```python
from build123d import *

# Parameters (mm, degrees)
EXTRUSION1_DEPTH           = 2.1
ESQUISSE2_R                = 5.85
EXTRUSION2_DEPTH           = 5.2
ESQUISSE3_R                = 1.75
EXTRUSION3_DEPTH           = 39.762384708
ESQUISSE4_R                = 3.15
EXTRUSION4_DEPTH           = 4
ESQUISSE5_R                = 2.95
EXTRUSION5_DEPTH           = 3.2
CHANFREIN2_SIZE            = 1.2
D_GAGEMENT_M21_D           = 1.8
R_P_TITION_LIN_AIRE1_COUNT = 6
R_P_TITION_LIN_AIRE1_PITCH = 3.2


with BuildPart() as part:
    # Esquisse1 → Extrusion1 (new body)
    with BuildSketch(Plane.XY):
        with BuildLine():
            Line((-0.179008677, 4.246228432), (30.191384159, 5.526556123))
            ThreePointArc((30.191384159, 5.526556123), (37.220312431, -1.486890222), (29.654324486, -7.917293686))
            Line((29.654324486, -7.917293686), (-0.51715736, -4.218417744))
            ThreePointArc((-0.51715736, -4.218417744), (-4.246612828, 0.169645193), (-0.179008677, 4.246228432))
        make_face()
    extrude(amount=EXTRUSION1_DEPTH)

    # Esquisse2 → Extrusion2 (add)
    with BuildSketch(Plane(origin=(0, 0, 0), x_dir=(-1, 0, 0), z_dir=(0, 0, -1))):
        with Locations(Location((-30.475692058, -1.217453739, 0), (0, 0, 180))):
            Circle(ESQUISSE2_R)
    extrude(amount=EXTRUSION2_DEPTH)

    # Esquisse3 → Extrusion3 (cut, through all)
    with BuildSketch(Plane(origin=(0, 0, -5.2), x_dir=(-1, 0, 0), z_dir=(0, 0, -1))):
        with Locations((-30.475692058, -1.217453739)):
            Circle(ESQUISSE3_R)
    extrude(amount=-EXTRUSION3_DEPTH, mode=Mode.SUBTRACT)

    # Esquisse4 → Extrusion4 (cut)
    with BuildSketch(Plane.XY.offset(2.1)):
        with Locations((30.475692058, -1.217453739)):
            Circle(ESQUISSE4_R)
    extrude(amount=-EXTRUSION4_DEPTH, mode=Mode.SUBTRACT)

    # Esquisse5 → Extrusion5 (cut)
    with BuildSketch(Plane(origin=(0, 0, -5.2), x_dir=(-1, 0, 0), z_dir=(0, 0, -1))):
        with Locations((-30.475692058, -1.217453739)):
            Circle(ESQUISSE5_R)
    extrude(amount=-EXTRUSION5_DEPTH, mode=Mode.SUBTRACT)

    # Chanfrein2
    chanfrein2_edges = [part.edges().sort_by_distance(p)[0] for p in [
        (24.625692058, -1.217453739, -5.2),
        (27.325692058, -1.217453739, 2.1),
    ]]
    chamfer(chanfrein2_edges, length=CHANFREIN2_SIZE)

    # D_gagement M21 (through all)
    with Locations(Plane(origin=(-0.55, 0, 2.1), x_dir=(1, 0, 0), z_dir=(0, 0, 1))):
        with Locations((0, 0)):
            d_gagement_m21 = Hole(D_GAGEMENT_M21_D / 2)

    # R_p_tition lin_aire1: D_gagement M21 ×6
    with Locations(*[Vector(0.9992309921094119, -0.0392100039280862, 0) * (i * R_P_TITION_LIN_AIRE1_PITCH) for i in range(1, R_P_TITION_LIN_AIRE1_COUNT)]):
        add(d_gagement_m21, mode=Mode.SUBTRACT)


solid = part.part
```
Input: part model. Units: mm. Frame: model coordinates. A direction names the side the tool comes from. Give positions to 0.01 mm unless a question says otherwise; leave off trailing zeros. Loops run counter-clockwise (first coordinate to the right, second up) from the corner with the lowest first, then second, coordinate; pieces in that order, holes last.
1) Line query: L1, parallel to Z at x = 5.5, y = -3.5; L2, parallel to Z at x = 34.5, y = 2.5; L3, parallel to X at y = -3.25, z = -3. Output: solid intervals per line, ascending.
A:
L1: z = 0 to 2.1
L2: z = -4.37 to 2.1
L3: x = 24.99 to 28.34, 32.61 to 35.96
2) Section query A-A on x = 12. Return the cut outline in (y, z).
A:
outline: (-5.75, 0) - (-1.37, 0) - (-1.37, 2.1) - (-5.75, 2.1) - close; (0.37, 0) - (4.76, 0) - (4.76, 2.1) - (0.37, 2.1) - close
3) Reachability of faces 1 (the cylindrical face through (27.75, -2.35, -3.62)), 2 (the flat face through (17, -1, 2.1)), 3 (the cylindrical face through (27.33, -1.08, -0.48)) from +Z, -Z, +X, -X, +Y, -Y: full face, straight path, thin tool, end or side. Return the list, or none.
A:
face 1: -Z
face 2: +Z, +X, -X, +Y, -Y
face 3: +Z
4) Mould query, pull axis Y, two halves, no side actions, for faces 4 (the cylindrical face through (16.1, -0.02, 1.04)), 5 (the flat face through (14.78, -6.094, 1.035)), 6 (the cylindrical face through (-4.25, 0.08, 1.04)), 7 (the cylindrical face through (5.014, -0.596, 1.035)). Classes: released by +Y, released by -Y, zero draft, split by the parting line, or undercut.
A:
face 4: undercut
face 5: released by -Y
face 6: split by the parting line
face 7: undercut
5) Contact query for flat-ended pins moving along their axis: pin 1 (2 mm diameter, centred on x = 11.5, z = 0.5, fed in from -Y); pin 2 (5 mm diameter, centred on x = 31.5, y = -1.5, fed in from +Z); pin 3 (4 mm diameter, centred on x = 16, z = -3, fed in from -Y); pin 4 (4 mm diameter, centred on x = 2, z = 0, fed in from +Y). Output: stop coordinate, or through.
A:
pin 1: stops at y = -5.81
pin 2: stops at z = 1.31
pin 3: passes through
pin 4: stops at y = 4.42
